Check sheet for the modelled part. Datum: model origin and axes. Units: mm. Give positions to 0.01 mm unless a question says otherwise; leave off trailing zeros. Write each loop counter-clockwise with the first axis right and the second up, starting at its lowest first coordinate (ties: lowest second). Pieces come first, ordered by that corner, then holes. Notation, with made-up numbers: (83, -10.75) -> (102, -10.75) arc R32 cw to (102, 24.25) -> close; hole circle Ø2 at (11.5, 83). An arc over 180 degrees is marked (long way). Use a Markdown table: item, result. Add a question column.
1. Gauge pin test, flat ends, axial feed: P1, Ø12, axis at y = 113.5, z = 1, coming from the -X side; P2, Ø3, axis at y = 67, z = 1, coming from the -X side; P3, Ø2.5, axis at x = 0, z = 0, coming from the +Y side; P4, Ø4, axis at x = 0.5, y = 174, coming from the +Z side. Record the tip position at first contact, or that the pin passes through.
2. Scan lines: probe 1 along X at (y, z) = (102.75, 0); probe 2 along Z at (x, y) = (-4.25, 105); probe 3 along Y at (x, z) = (4, 1.75). Record each from-to range of solid material in increasing order. Write a range as [from, to].
3. Cross-section at B-B (z = 0). Enter the section's corners in (x, y), then the cut area to 3 significant figures.
4. Cross-section at A-A (x = 0). Enter the section's corners in (y, z).
5. Cross-section at C-C (y = 78). Count the separate pieces of the cut face and the enclosed holes in it, then the cut area to 3 significant figures.
from build123d import *

# Parameters (mm, degrees)
SKETCH1_W           = 20
SKETCH1_H           = 20
EXTRUDE1_DEPTH      = 200
SKETCH2_R           = 2.266666667
SKETCH2_W           = 1.866666667
SKETCH2_H           = 1.866666667
EXTRUDE2_DEPTH      = 201.499376558
FILLET1_R           = 1.333333333
SKETCH_1_R          = 2.5
CUT_EXTRUDE_1_DEPTH = 202.246117975


with BuildPart() as part:
    # Sketch1 → Extrude1 (new body)
    with BuildSketch(Plane(origin=(0, 0, 0), x_dir=(1, 0, 0), z_dir=(0, 1, 0))):
        Rectangle(SKETCH1_W, SKETCH1_H)
    extrude(amount=EXTRUDE1_DEPTH)

    # Sketch2 → Extrude2 (cut, through all)
    with BuildSketch(Plane(origin=(0, 200, 0), x_dir=(1, 0, 0), z_dir=(0, 1, 0))):
        with Locations(Location((0, 0, 0), (0, 0, 270))):
            Circle(SKETCH2_R)
        Polygon((8.666666667, 3), (11.333333333, 3), (11.333333333, -3), (8.666666667, -3), (8.666666667, -5.466666667), (6.409475708, -5.466666667), (4.133333333, -3.190524292), (4.133333333, 3.190524292), (6.409475708, 5.466666667), (8.666666667, 5.466666667), align=None)
        with Locations((7.733333334, 7.733333334)):
            Rectangle(SKETCH2_W, SKETCH2_H)
        Polygon((-3.190524292, 4.133333333), (-5.466666667, 6.409475708), (-5.466666667, 8.666666667), (-3, 8.666666667), (-3, 11.333333333), (3, 11.333333333), (3, 8.666666667), (5.466666667, 8.666666667), (5.466666667, 6.409475708), (3.190524292, 4.133333333), align=None)
        with Locations((7.733333334, -7.733333334)):
            Rectangle(SKETCH2_W, SKETCH2_H)
        with Locations((-7.733333334, 7.733333334)):
            Rectangle(SKETCH2_W, SKETCH2_H)
        with Locations((-7.733333334, -7.733333334)):
            Rectangle(SKETCH2_W, SKETCH2_H)
        Polygon((-6.409475708, -5.466666667), (-8.666666667, -5.466666667), (-8.666666667, -3), (-11.333333333, -3), (-11.333333333, 3), (-8.666666667, 3), (-8.666666667, 5.466666667), (-6.409475708, 5.466666667), (-4.133333333, 3.190524292), (-4.133333333, -3.190524292), align=None)
        Polygon((3.190524292, -4.133333333), (-3.190524292, -4.133333333), (-5.466666667, -6.409475708), (-5.466666667, -8.666666667), (-3, -8.666666667), (-3, -11.333333333), (3, -11.333333333), (3, -8.666666667), (5.466666667, -8.666666667), (5.466666667, -6.409475708), align=None)
    extrude(amount=-EXTRUDE2_DEPTH, mode=Mode.SUBTRACT)

    # Fillet1
    fillet1_edges = [part.edges().sort_by_distance(p)[0] for p in [
        (10, 100, 10),
        (-10, 100, 10),
        (-10, 100, -10),
        (10, 100, -10),
    ]]
    fillet(fillet1_edges, radius=FILLET1_R)

    # Sketch 1 → Cut-Extrude 1 (cut, through all)
    with BuildSketch(Plane(origin=(10, 0, 0), x_dir=(0, 0, -1), z_dir=(1, 0, 0))):
        with Locations((0, 93)):
            Circle(SKETCH_1_R)
        with Locations((0, 107)):
            Circle(SKETCH_1_R)
    extrude(amount=-CUT_EXTRUDE_1_DEPTH, mode=Mode.SUBTRACT)


solid = part.part
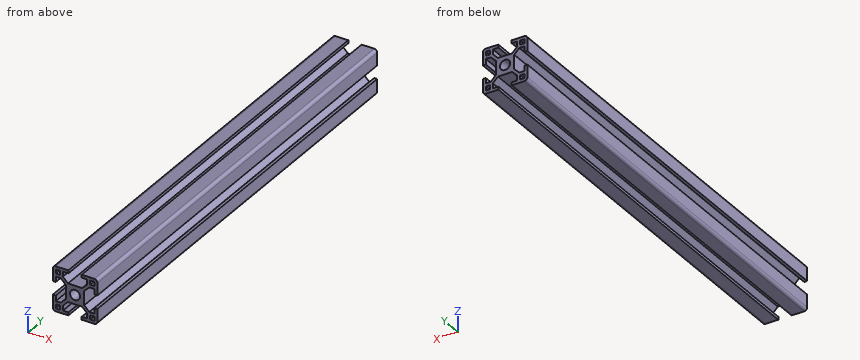
Worked answers:
| question | item | result |
|---|---|---|
| 1 | P1 | stops at x = -10 |
| 1 | P2 | stops at x = -4.13 |
| 1 | P3 | passes through |
| 1 | P4 | stops at z = 4.13 |
| 2 | probe 1 | x = [-4.13, -2.27], [2.27, 4.13] |
| 2 | probe 2 | z = [-10, -8.67], [-5.19, -3.31], [3.31, 5.19], [8.67, 10] |
| 2 | probe 3 | y = [0, 91.21], [94.79, 105.21], [108.79, 200] |
| 3 | outline | (-4.13, 0) -> (-2.27, 0) -> (-2.27, 90.5) -> (-4.13, 90.5) -> close; (-4.13, 95.5) -> (-2.27, 95.5) -> (-2.27, 104.5) -> (-4.13, 104.5) -> close; (-4.13, 109.5) -> (-2.27, 109.5) -> (-2.27, 200) -> (-4.13, 200) -> close; (2.27, 0) -> (4.13, 0) -> (4.13, 90.5) -> (2.27, 90.5) -> close; (2.27, 95.5) -> (4.13, 95.5) -> (4.13, 104.5) -> (2.27, 104.5) -> close; (2.27, 109.5) -> (4.13, 109.5) -> (4.13, 200) -> (2.27, 200) -> close |
| 3 | area | 709 mm² |
| 4 | outline | (0, -4.13) -> (200, -4.13) -> (200, -2.27) -> (108.05, -2.27) arc R2.5 cw to (105.95, -2.27) -> (94.05, -2.27) arc R2.5 cw to (91.95, -2.27) -> (0, -2.27) -> close; (0, 2.27) -> (91.95, 2.27) arc R2.5 cw to (94.05, 2.27) -> (105.95, 2.27) arc R2.5 cw to (108.05, 2.27) -> (200, 2.27) -> (200, 4.13) -> (0, 4.13) -> close |
| 5 | separate pieces | 1 |
| 5 | enclosed holes | 5 |
| 5 | area | 159 mm² |
